Source: CAD feature listing. Evaluate the final solid. Frame: model axes, mm. A direction names the side the tool comes from. Coordinates: 2 decimals unless noted, no trailing zeros. Write each loop counter-clockwise with the first axis right and the second up, starting at its lowest first coordinate (ties: lowest second). Pieces come first, ordered by that corner, then holes. Notation, with made-up numbers: (54, 66.5) -> (73, 66.5) arc R16 ccw to (73, 73.5) -> close; hole circle Ø5 at (85.5, 29). An arc over 180 degrees is marked (long way). Write item = value, one per line.
from build123d import *

# Parameters (mm, degrees)
FILLET_1_R = 0.2


with BuildPart() as part:
    # 草图1 → 旋转1 (revolve)
    with BuildSketch(Plane.XY, mode=Mode.PRIVATE) as revolve_1_sk:
        Polygon((2.5, 4), (2.5, 0), (3.3, 0), (3.3, 0.5), (5.6, 0.5), (5.6, 0), (7.5, 0), (7.5, 1), (6.5, 1), (6.5, 4), (5.6, 4), (5.6, 3.5), (3.3, 3.5), (3.3, 4), align=None)
    revolve(revolve_1_sk.sketch.rotate(Axis((0, 5.412170411, 0), (0, -1, 0)), 90), axis=Axis((0, 5.412170411, 0), (0, -1, 0)))

    # 圆角1
    fillet_1_edges = [part.edges().sort_by_distance(p)[0] for p in [
        (0, 0, -2.5),
        (0, 4, -2.5),
        (0, 4, -6.5),
        (0, 0, -7.5),
    ]]
    fillet(fillet_1_edges, radius=FILLET_1_R)


solid = part.part
1) First-contact query: pin 1 Ø1.5 at (x, y) = (-6, 3.5) entering from -Z; pin 2 Ø1.5 at (y, z) = (1.5, 4.5) entering from +X; pin 3 Ø3 at (x, z) = (0, 0) entering from +Y; pin 4 Ø1.5 at (y, z) = (3, -0.5) entering from -X. Flat tips, straight axial feed; report the tip coordinate or a pass-through.
Answer block:
pin_1 = -3.83
pin_2 = 6.38
pin_3 = through
pin_4 = -6.5
2) Cut plane A-A, the plane y = 2.5. Output: boundary loops of the cut face in (x, z), and give its area (3 significant figures).
Answer block:
outline = circle Ø13 at (0, 0); hole circle Ø5 at (0, 0)
area = 113 mm2
3) Reachability of faces 4 (the cylindrical face through (-0.246, 0.246, -5.595)), 5 (the flat face through (-3, 1, -6)), 6 (the flat face through (0, 4, -6)) from +Z, -Z, +X, -X, +Y, -Y: full face, straight path, thin tool, end or side. Return the list, or none.
Answer block:
face_4 = -Y
face_5 = +Y
face_6 = +Z, -Z, +X, -X, +Y
4) Pull-direction query (X, two-part tool) for faces 1 (the cylindrical face through (3.955, 2.42, -5.158)), 2 (the flat face through (0, 4, -3)), 3 (the cylindrical face through (-0.246, 3.746, -5.595)); classes: +X half, -X half, draft (parallel to the pull), parting line (faces both ways), or undercut.
Answer block:
face_1 = parting line
face_2 = draft
face_3 = undercut
5) Material intervals for probe 1 along X at (y, z) = (3, 0); probe 2 along X at (y, z) = (3.85, 0); probe 3 along Y at (x, z) = (-1.5, 4), sorted ascending. Write a range as [from, to].
Answer block:
probe_1 = [-6.5, -2.5], [2.5, 6.5]
probe_2 = [-6.49, -5.6], [-3.3, -2.51], [2.51, 3.3], [5.6, 6.49]
probe_3 = [0.5, 3.5]
